Could you check a few things on this model? Use its own coordinates, in mm. Give positions to 0.01 mm unless a question says otherwise; leave off trailing zeros. Write each loop counter-clockwise with the first axis right and the second up, starting at its lowest first coordinate (ties: lowest second). Pieces come first, ordered by that corner, then holes. Notation, with made-up numbers: (-39, 40) - (-17, 40) arc R22 cw to (-17, 78) - close; hole circle Ø5 at (12, 48). An arc over 180 degrees is marked (long way). Answer in a Markdown table with one row per item.
from build123d import *

# Parameters (mm, degrees)
ESBO_O2_R                = 3.3
ESBO_O2_R_2              = 2.3
RESSALTO_EXTRUS_O1_DEPTH = 4.8
RESSALTO_EXTRUS_O2_START = -1.5
ESBO_O3_R                = 0.5
RESSALTO_EXTRUS_O2_DEPTH = 1.5


with BuildPart() as part:
    # Esboço2 → Ressalto-extrusão1 (new body)
    with BuildSketch(Plane(origin=(0, 0, 0), x_dir=(1, 0, 0), z_dir=(0, 1, 0))):
        with Locations(Location((0, 0, 0), (0, 0, 270))):
            Circle(ESBO_O2_R)
        with Locations(Location((0, 0, 0), (0, 0, 270))):
            Circle(ESBO_O2_R_2, mode=Mode.SUBTRACT)
    extrude(amount=RESSALTO_EXTRUS_O1_DEPTH)

    # Esboço3 → Ressalto-extrusão2 (add)
    # profile 1 of 2: a face of its own
    with BuildSketch(Plane(origin=(0, 4.8, 0), x_dir=(1, 0, 0), z_dir=(0, 1, 0)).offset(RESSALTO_EXTRUS_O2_START)):
        with BuildLine():
            Line((14.2, 2), (1.374772708, 3))
            ThreePointArc((1.374772708, 3), (2.777296342, 1.782308904), (3.3, 0))
            ThreePointArc((3.3, 0), (2.777296342, -1.782308904), (1.374772708, -3))
            Line((1.374772708, -3), (14.2, -2))
            ThreePointArc((14.2, -2), (16.2, 0), (14.2, 2))
        make_face()
        with Locations(Location((4.2, 0, 0), (0, 0, 270))):
            Circle(ESBO_O3_R, mode=Mode.SUBTRACT)
        with Locations(Location((6.2, 0, 0), (0, 0, 270))):
            Circle(ESBO_O3_R, mode=Mode.SUBTRACT)
        with Locations(Location((8.2, 0, 0), (0, 0, 270))):
            Circle(ESBO_O3_R, mode=Mode.SUBTRACT)
        with Locations(Location((10.2, 0, 0), (0, 0, 270))):
            Circle(ESBO_O3_R, mode=Mode.SUBTRACT)
        with Locations(Location((12.2, 0, 0), (0, 0, 270))):
            Circle(ESBO_O3_R, mode=Mode.SUBTRACT)
        with Locations(Location((14.2, 0, 0), (0, 0, 270))):
            Circle(ESBO_O3_R, mode=Mode.SUBTRACT)
    # profile 2 of 2: a face of its own
    with BuildSketch(Plane(origin=(0, 4.8, 0), x_dir=(1, 0, 0), z_dir=(0, 1, 0)).offset(RESSALTO_EXTRUS_O2_START)):
        with BuildLine():
            ThreePointArc((-1.374772708, -3), (-3.3, 0), (-1.374772708, 3))
            Line((-1.374772708, 3), (-14.2, 2))
            ThreePointArc((-14.2, 2), (-16.2, 0), (-14.2, -2))
            Line((-14.2, -2), (-1.374772708, -3))
        make_face()
        with Locations(Location((-14.2, 0, 0), (0, 0, 270))):
            Circle(ESBO_O3_R, mode=Mode.SUBTRACT)
        with Locations(Location((-12.2, 0, 0), (0, 0, 270))):
            Circle(ESBO_O3_R, mode=Mode.SUBTRACT)
        with Locations(Location((-10.2, 0, 0), (0, 0, 270))):
            Circle(ESBO_O3_R, mode=Mode.SUBTRACT)
        with Locations(Location((-8.2, 0, 0), (0, 0, 270))):
            Circle(ESBO_O3_R, mode=Mode.SUBTRACT)
        with Locations(Location((-6.2, 0, 0), (0, 0, 270))):
            Circle(ESBO_O3_R, mode=Mode.SUBTRACT)
        with Locations(Location((-4.2, 0, 0), (0, 0, 270))):
            Circle(ESBO_O3_R, mode=Mode.SUBTRACT)
    extrude(amount=RESSALTO_EXTRUS_O2_DEPTH)


solid = part.part
1) We'd pull the mould along Z, two halves only. Please class faces 1 (the face through (-7.704, 4.04, -0.065)), 2 (the face through (16.2, 4, 0)), 3 (the face through (7.698, 4.04, 2.507)): +Z half, -Z half, draft (parallel to the pull), parting line (faces both ways), or undercut.
Check values:
| item | result |
|---|---|
| face 1 | undercut |
| face 2 | parting line |
| face 3 | +Z half |
2) Imagine slicing it at C-C (y = 1.2). List the corners of the cut face in (x, z) for me, then the cut area to 3 significant figures.
Check values:
| item | result |
|---|---|
| outline | circle Ø6.6 at (0, 0); hole circle Ø4.6 at (0, 0) |
| area | 17.6 mm2 |
3) Imagine slicing it at B-B (z = 1.25). List the corners of the cut face in (x, y) for me.
Check values:
| item | result |
|---|---|
| outline | (-15.76, 3.3) - (-3.05, 3.3) - (-3.05, 0) - (-1.93, 0) - (-1.93, 4.8) - (-15.76, 4.8) - close; (1.93, 0) - (3.05, 0) - (3.05, 3.3) - (15.76, 3.3) - (15.76, 4.8) - (1.93, 4.8) - close |
4) Imagine slicing it at A-A (x = 0). List the corners of the cut face in (y, z) for me.
Check values:
| item | result |
|---|---|
| outline | (0, -3.3) - (4.8, -3.3) - (4.8, -2.3) - (0, -2.3) - close; (0, 2.3) - (4.8, 2.3) - (4.8, 3.3) - (0, 3.3) - close |
5) If I drill on line 1 (Y direction, x = -14, z = 1.75); line 2 (X direction, y = 2, z = -0.25); line 3 (X direction, y = 3.9, z = 1.25), over which ranges is the centre line in solid material (lowest first)?
Check values:
| item | result |
|---|---|
| line 1 | y = 3.3 to 4.8 |
| line 2 | x = -3.29 to -2.29, 2.29 to 3.29 |
| line 3 | x = -15.76 to -1.93, 1.93 to 15.76 |
6) Will these pins go through, and if not, where does the flat tip stop? P1, Ø3, axis at x = 0, z = 0, coming from the -Y side; P2, Ø1.5, axis at x = 3.5, y = 4.5, coming from the +Z side.
Check values:
| item | result |
|---|---|
| P1 | passes through |
| P2 | stops at z = 2.89 |
7) Imagine slicing it at D-D (z = 0). State how many separate pieces and enclosed holes the cut face has, then the cut area to 3 significant figures.
Check values:
| item | result |
|---|---|
| separate pieces | 14 |
| enclosed holes | 0 |
| area | 30.3 mm2 |
